Verification items for the finished model (mm, model axes). A direction names the side the tool comes from. Give positions to 0.01 mm unless a question says otherwise; leave off trailing zeros. Loops run counter-clockwise (first coordinate to the right, second up) from the corner with the lowest first, then second, coordinate; pieces in that order, holes last. Notation, with made-up numbers: (-9.5, 28.5) -> (7.5, 28.5) arc R12 cw to (7.5, 48.5) -> close; hole circle Ø8 at (46, -32.75). An arc over 180 degrees is marked (long way). Answer in a Markdown table with one row per item. Add a question column.
Q1. Section check D-D on z = -9. Enter the section's corners in (x, y), and give its area (3 significant figures).
Q2. Section check B-B on x = -6. Enter the section's corners in (y, z).
Q3. Material ranges on probe 1 along Y at (x, z) = (-5.65, 25); probe 2 along Y at (x, z) = (13, 4.95); probe 3 along X at (y, z) = (8.5, 26.5), recorded low to high.
Q4. Set-up check for faces 5 (the face through (18, 0, -18)), 6 (the face through (11.05, 1, 38)), 7 (the face through (-2, 0, 14)), 8 (the face through (19.1, 3, 24)), 9 (the face through (7.95, 1, 38)): record each of +Z, -Z, +X, -X, +Y, -Y from which the full face is reachable in a straight line by a thin tool's end or side.
Q5. Release check for a two-part mould opening along Y. For faces 1 (the face through (9, 11.25, 17)), 2 (the face through (21.5, 0, -6)), 3 (the face through (-6.364, 0.24, 24.237)), 4 (the face through (9.633, 7.384, 5.264)) record: pulls with the +Y half, pulls with the -Y half, needs draft (parallel to the pull), parting line crosses it, or undercut.
Q6. Gauge pin test, flat ends, axial feed: P1, Ø8, axis at y = -5.5, z = 10.5, coming from the -X side; P2, Ø0.8, axis at x = 20, z = -6, coming from the -Y side; P3, Ø8, axis at y = -0.5, z = -15, coming from the -X side. Record the tip position at first contact, or that the pin passes through.
Q7. Section check A-A on z = 39.6. Enter the section's corners in (x, y), and give its area (3 significant figures).
Q8. Section check C-C on z = 13.75. Enter the section's corners in (x, y), and give its area (3 significant figures).
```python
from build123d import *

# Parameters (mm, degrees)
SKETCH1_W                 = 37
SKETCH1_H                 = 22.5
BOSS_EXTRUDE1_DEPTH       = 19
SKETCH2_W                 = 3.1
SKETCH2_H                 = 5.3
BOSS_EXTRUDE2_DEPTH       = 5.2
SKETCH3_R                 = 1.35
CUT_EXTRUDE1_DEPTH        = 12.05
FILLET1_R                 = 3.5
SKETCH4_R                 = 3.6
BOSS_EXTRUDE3_DEPTH       = 0.1
SKETCH5_R                 = 3.6
BOSS_EXTRUDE4_DEPTH       = 0.1
SKETCH6_R                 = 2.7
BOSS_EXTRUDE5_DEPTH       = 8.9
SKETCH7_R                 = 2.7
BOSS_EXTRUDE6_DEPTH       = 8.9
FILLET2_R                 = 0.5
CUT_EXTRUDE2_DEPTH        = 8.2
CUT_EXTRUDE3_DEPTH        = 8.2
M2X0_4_TAPPED_HOLE1_D     = 1.6
M2X0_4_TAPPED_HOLE1_DEPTH = 5.2
M2X0_4_TAPPED_HOLE1_TIP   = 0.480688495
M2X0_4_TAPPED_HOLE2_D     = 1.6
M2X0_4_TAPPED_HOLE2_DEPTH = 5.2
M2X0_4_TAPPED_HOLE2_TIP   = 0.480688495
SKETCH16_R                = 1.95
BOSS_EXTRUDE7_DEPTH       = 2
BOSS_EXTRUDE8_DEPTH       = 11.5
SKETCH18_W                = 3.5
SKETCH18_H                = 5.2
BOSS_EXTRUDE9_DEPTH       = 2.5
SKETCH19_W                = 3.5
SKETCH19_H                = 5.2
BOSS_EXTRUDE10_DEPTH      = 2.5
BOSS_EXTRUDE11_DEPTH      = 13.5
FILLET3_R                 = 1.7
BOSS_EXTRUDE12_DEPTH      = 2
SKETCH25_R                = 1.45
CUT_EXTRUDE5_DEPTH        = 29


with BuildPart() as part:
    # Sketch1 → Boss-Extrude1 (new body)
    with BuildSketch(Plane(origin=(0, 0, 0), x_dir=(0, 0, -1), z_dir=(1, 0, 0))):
        with Locations((-18.5, 0)):
            Rectangle(SKETCH1_W, SKETCH1_H)
    extrude(amount=BOSS_EXTRUDE1_DEPTH)

    # Sketch2 → Boss-Extrude2 (add)
    with BuildSketch(Plane.XY.offset(37)):
        with Locations((9.5, 0)):
            Rectangle(SKETCH2_W, SKETCH2_H)
    extrude(amount=BOSS_EXTRUDE2_DEPTH)

    # Sketch3 → Cut-Extrude1 (cut, through all)
    with BuildSketch(Plane(origin=(11.05, 0, 0), x_dir=(0, 0, -1), z_dir=(1, 0, 0))):
        with Locations((-39.6, 0)):
            Circle(SKETCH3_R)
    extrude(amount=-CUT_EXTRUDE1_DEPTH, mode=Mode.SUBTRACT)

    # Fillet1
    fillet1_edges = [part.edges().sort_by_distance(p)[0] for p in [
        (9.5, -11.25, 37),
        (9.5, 11.25, 37),
    ]]
    fillet(fillet1_edges, radius=FILLET1_R)

    # Sketch4 → Boss-Extrude3 (add)
    with BuildSketch(Plane(origin=(19, 0, 0), x_dir=(0, 0, -1), z_dir=(1, 0, 0))):
        with Locations((-25, 0)):
            Circle(SKETCH4_R)
    extrude(amount=BOSS_EXTRUDE3_DEPTH)

    # Sketch5 → Boss-Extrude4 (add)
    with BuildSketch(Plane.ZY):
        with Locations((25, 0)):
            Circle(SKETCH5_R)
    extrude(amount=BOSS_EXTRUDE4_DEPTH)

    # Sketch6 → Boss-Extrude5 (add)
    with BuildSketch(Plane(origin=(19.1, 0, 0), x_dir=(0, 0, -1), z_dir=(1, 0, 0))):
        with Locations((-25, 0)):
            Circle(SKETCH6_R)
    extrude(amount=BOSS_EXTRUDE5_DEPTH)

    # Sketch7 → Boss-Extrude6 (add)
    with BuildSketch(Plane.ZY.offset(0.1)):
        with Locations((25, 0)):
            Circle(SKETCH7_R)
    extrude(amount=BOSS_EXTRUDE6_DEPTH)

    # Fillet2
    fillet2_edges = [part.edges().sort_by_distance(p)[0] for p in [
        (9.5, 2.65, 37),
        (9.5, -2.65, 37),
    ]]
    fillet(fillet2_edges, radius=FILLET2_R)

    # Sketch8 → Cut-Extrude2 (cut)
    with BuildSketch(Plane(origin=(28, 0, 0), x_dir=(0, 0, -1), z_dir=(1, 0, 0))):
        with BuildLine():
            Line((-26.8, -2.01246118), (-26.8, 2.01246118))
            ThreePointArc((-26.8, 2.01246118), (-27.7, 0), (-26.8, -2.01246118))
        make_face()
        with BuildLine():
            ThreePointArc((-22.3, 0), (-22.535248491, 1.102270384), (-23.2, 2.01246118))
            Line((-23.2, 2.01246118), (-23.2, -2.01246118))
            ThreePointArc((-23.2, -2.01246118), (-22.535248491, -1.102270384), (-22.3, 0))
        make_face()
    extrude(amount=-CUT_EXTRUDE2_DEPTH, mode=Mode.SUBTRACT)

    # Sketch9 → Cut-Extrude3 (cut)
    with BuildSketch(Plane.ZY.offset(9)):
        with BuildLine():
            Line((23.2, -2.01246118), (23.2, 2.01246118))
            ThreePointArc((23.2, 2.01246118), (22.3, 0), (23.2, -2.01246118))
        make_face()
        with BuildLine():
            ThreePointArc((27.7, 0), (27.464751509, 1.102270384), (26.8, 2.01246118))
            Line((26.8, 2.01246118), (26.8, -2.01246118))
            ThreePointArc((26.8, -2.01246118), (27.464751509, -1.102270384), (27.7, 0))
        make_face()
    extrude(amount=-CUT_EXTRUDE3_DEPTH, mode=Mode.SUBTRACT)

    # M2x0.4 Tapped Hole1
    with Locations(Plane(origin=(28, 0, 0), x_dir=(0, 0, -1), z_dir=(1, 0, 0))):
        with Locations((-25, 0)):
            Hole(M2X0_4_TAPPED_HOLE1_D / 2, depth=M2X0_4_TAPPED_HOLE1_DEPTH)
            with Locations((0, 0, -(M2X0_4_TAPPED_HOLE1_DEPTH + M2X0_4_TAPPED_HOLE1_TIP / 2))):  # 118° drill point
                Cone(0, M2X0_4_TAPPED_HOLE1_D / 2, M2X0_4_TAPPED_HOLE1_TIP, mode=Mode.SUBTRACT)

    # M2x0.4 Tapped Hole2
    with Locations(Plane.ZY.offset(9)):
        with Locations((25, 0)):
            Hole(M2X0_4_TAPPED_HOLE2_D / 2, depth=M2X0_4_TAPPED_HOLE2_DEPTH)
            with Locations((0, 0, -(M2X0_4_TAPPED_HOLE2_DEPTH + M2X0_4_TAPPED_HOLE2_TIP / 2))):  # 118° drill point
                Cone(0, M2X0_4_TAPPED_HOLE2_D / 2, M2X0_4_TAPPED_HOLE2_TIP, mode=Mode.SUBTRACT)

    # Sketch16 → Boss-Extrude7 (add)
    with BuildSketch(Plane.ZY):
        with Locations((13.75, 0)):
            Circle(SKETCH16_R)
    extrude(amount=BOSS_EXTRUDE7_DEPTH)

    # Sketch17 → Boss-Extrude8 (add)
    with BuildSketch(Plane(origin=(0, 0, 0), x_dir=(-1, 0, 0), z_dir=(0, 0, -1))):
        with BuildLine():
            Line((-19, 6.025985397), (-19, -6.025985397))
            ThreePointArc((-19, -6.025985397), (-10.560588754, -11.199895156), (-1.3, -7.7021101))
            Line((-1.3, -7.7021101), (-1.3, 7.7021101))
            ThreePointArc((-1.3, 7.7021101), (-10.560588754, 11.199895156), (-19, 6.025985397))
        make_face()
    extrude(amount=BOSS_EXTRUDE8_DEPTH)

    # Sketch18 → Boss-Extrude9 (add)
    with BuildSketch(Plane(origin=(19, 0, 0), x_dir=(0, 0, -1), z_dir=(1, 0, 0))):
        with Locations((5.75, 0)):
            Rectangle(SKETCH18_W, SKETCH18_H)
    extrude(amount=BOSS_EXTRUDE9_DEPTH)

    # Sketch19 → Boss-Extrude10 (add)
    with BuildSketch(Plane.ZY.offset(-1.3)):
        with Locations((-5.75, 0)):
            Rectangle(SKETCH19_W, SKETCH19_H)
    extrude(amount=BOSS_EXTRUDE10_DEPTH)

    # Sketch20 → Boss-Extrude11 (add)
    with BuildSketch(Plane(origin=(0, 0, -11.5), x_dir=(-1, 0, 0), z_dir=(0, 0, -1))):
        with BuildLine():
            Line((-18, 5.728219619), (-18, -5.728219619))
            ThreePointArc((-18, -5.728219619), (-10.518083587, -10.199313987), (-2.3, -7.295375247))
            Line((-2.3, -7.295375247), (-2.3, 7.295375247))
            ThreePointArc((-2.3, 7.295375247), (-10.518083587, 10.199313987), (-18, 5.728219619))
        make_face()
    extrude(amount=BOSS_EXTRUDE11_DEPTH)

    # Fillet3
    fillet3_edges = [part.edges().sort_by_distance(p)[0] for p in [
        (10.518083587, 10.199313987, -25),
        (10.518083587, -10.199313987, -25),
    ]]
    fillet(fillet3_edges, radius=FILLET3_R)

    # Sketch21 → Boss-Extrude12 (add)
    with BuildSketch(Plane(origin=(0, 0, -25), x_dir=(-1, 0, 0), z_dir=(0, 0, -1))):
        with BuildLine():
            Line((-5.5, -3), (-5.5, 3))
            ThreePointArc((-5.5, 3), (-14.5, 0), (-5.5, -3))
        make_face()
    extrude(amount=BOSS_EXTRUDE12_DEPTH)

    # Sketch25 → Cut-Extrude5 (cut, through all)
    with BuildSketch(Plane(origin=(19, 0, 0), x_dir=(0, 0, -1), z_dir=(1, 0, 0))):
        with Locations((-4.95, 8.8)):
            Circle(SKETCH25_R)
        with Locations((-4.95, -8.8)):
            Circle(SKETCH25_R)
    extrude(amount=-CUT_EXTRUDE5_DEPTH, mode=Mode.SUBTRACT)


solid = part.part
```
Taken from the geometry:
| question | item | result |
|---|---|---|
| 1 | outline | (1.3, -7.7) arc R11.25 ccw to (19, -6.03) -> (19, 6.03) arc R11.25 ccw to (1.3, 7.7) -> close |
| 1 | area | 351 mm² |
| 2 | outline | (-2.01, 23.2) -> (2.01, 23.2) arc R2.7 ccw to (2.01, 26.8) -> (-2.01, 26.8) arc R2.7 ccw to start; hole circle Ø1.6 at (0, 25) |
| 3 | probe 1 | y = -2.7 to -0.8, 0.8 to 2.7 |
| 3 | probe 2 | y = -11.25 to -10.25, -7.35 to 7.35, 10.25 to 11.25 |
| 3 | probe 3 | x = 0 to 19 |
| 4 | face 5 | -Z, +X, +Y, -Y |
| 4 | face 6 | +Z, +X, +Y, -Y |
| 4 | face 7 | -Z, -X, +Y, -Y |
| 4 | face 8 | +X |
| 4 | face 9 | +Z, -X, +Y, -Y |
| 5 | face 1 | pulls with the +Y half |
| 5 | face 2 | needs draft |
| 5 | face 3 | undercut |
| 5 | face 4 | undercut |
| 6 | P1 | stops at x = 0 |
| 6 | P2 | stops at y = -2.6 |
| 6 | P3 | stops at x = 1.3 |
| 7 | outline | (7.95, -2.65) -> (11.05, -2.65) -> (11.05, -1.35) -> (7.95, -1.35) -> close; (7.95, 1.35) -> (11.05, 1.35) -> (11.05, 2.65) -> (7.95, 2.65) -> close |
| 7 | area | 8.06 mm² |
| 8 | outline | (-2, -1.95) -> (0, -1.95) -> (0, -11.25) -> (19, -11.25) -> (19, 11.25) -> (0, 11.25) -> (0, 1.95) -> (-2, 1.95) -> close |
| 8 | area | 435 mm² |
